Model file for the job. Use its own axes, mm. Face numbers are marked on the shaded views. A direction names the side the tool comes from. Round coordinates to 2 decimals unless told otherwise and drop trailing zeros. Order: outer loops, then holes, each group sorted by start corner. A loop starts at its lowest first (then second) coordinate and runs counter-clockwise, first axis right, second up. Notation, with made-up numbers: (-37, -36) - (12, -36) arc R19 ccw to (12, -13) - close; hole circle Ø6 at (-36, 88.5). An arc over 180 degrees is marked (long way). Put each result on its own line as item: value. Start each with the question number.
Item 1: Saw through at A-A on y = 19.5. State how many separate pieces and enclosed holes the cut face has, plus the area to 3 significant figures.
Item 2: Saw through at D-D on z = 19.3. List the corners of the cut face in (x, y), plus the area to 3 significant figures.
Item 3: Probe probe 1 along Z at (x, y) = (36.5, -3.5); probe 2 along X at (y, z) = (-1.5, -38.7); probe 3 along X at (y, z) = (18.5, -33). List the from-to ranges inside material, lowest first.
Item 4: Mould opens along Z. For the marked faces 1, 2, 3 and 4 say: pulls with the +Z half, pulls with the -Z half, needs draft (parallel to the pull), parting line crosses it, or undercut.
Item 5: Saw through at C-C on x = 3.5. List the corners of the cut face in (y, z).
Item 6: Which spindle directions (+Z, -Z, +X, -X, +Y, -Y) get a long thin tool onto all of the face, cutting with end or side? Do the marked faces 5, 6, 7 and 8. Say none if no direction does.
Item 7: Pin check, flat tips, straight feed: pin 1 Ø2 at (y, z) = (8.5, 15) entering from -X; pin 2 Ø5 at (x, y) = (-63.5, -12) entering from -Z; pin 3 Ø13 at (x, z) = (36, -24.5) entering from +Y. Stop position of each tip, or through.
```python
from build123d import *

# Parameters (mm, degrees)
EXTRUDE_1_DEPTH     = 16
F_1_0MM_1_D         = 3.6
F_1_0MM_2_D         = 3.6
SKETCH_8_W          = 86.7
SKETCH_8_H          = 16
EXTRUDE_2_DEPTH     = 21.2
SKETCH_9_W          = 86.7
SKETCH_9_H          = 10.4
EXTRUDE_3_DEPTH     = 9.7
SKETCH_15_W         = 20.6
SKETCH_15_H         = 2
EXTRUDE_8_DEPTH     = 13.5
SKETCH_16_W         = 20.6
SKETCH_16_H         = 2
EXTRUDE_9_DEPTH     = 10.5
SKETCH_19_W         = 51.4
SKETCH_19_H         = 10.4
EXTRUDE_10_DEPTH    = 50
SKETCH_25_W         = 50
SKETCH_25_H         = 10.4
EXTRUDE_11_DEPTH    = 45
EXTRUDE_12_DEPTH    = 32
CUT_EXTRUDE_1_DEPTH = 5
SKETCH_29_W         = 51.4
SKETCH_29_H         = 10.402970243
EXTRUDE_13_DEPTH    = 40
SKETCH_32_W         = 40
SKETCH_32_H         = 10.402970243
EXTRUDE_14_DEPTH    = 10
SKETCH_33_W         = 40
SKETCH_33_H         = 10.402970243
EXTRUDE_15_DEPTH    = 10
SKETCH_34_R         = 3
EXTRUDE_16_DEPTH    = 18
F_1_0MM_3_D         = 3.6
F_1_0MM_4_D         = 3.6
FILLET_1_R          = 10
FILLET_2_R          = 10
SKETCH_40_W         = 6
SKETCH_40_H         = 4
EXTRUDE_17_DEPTH    = 11.5
SKETCH_42_W         = 6
SKETCH_42_H         = 19.4
EXTRUDE_18_DEPTH    = 2
SKETCH_46_W         = 60.1
SKETCH_46_H         = 4
EXTRUDE_19_DEPTH    = 2


with BuildPart() as part:
    # 草图1 → 凸台-拉伸1 (new body)
    with BuildSketch(Plane.XY):
        Polygon((-21.523113208, 25.59839861), (-42.123113208, 25.59839861), (-42.123113208, 5.59839861), (44.576886792, 5.59839861), (44.576886792, 25.59839861), (23.976886792, 25.59839861), (23.976886792, 13.12839861), (-21.523113208, 13.12839861), align=None)
    extrude_1 = extrude(amount=EXTRUDE_1_DEPTH)

    # Ø1.0mm 暗销孔1 (through all)
    with Locations(Plane(origin=(0, 25.59839861, 0), x_dir=(1, 0, 0), z_dir=(0, 1, 0))):
        with Locations((36.576886792, -8)):
            f_1_0mm_1 = Hole(F_1_0MM_1_D / 2)

    # Ø1.0mm 暗销孔2 (through all)
    with Locations(Plane(origin=(0, 25.59839861, 0), x_dir=(1, 0, 0), z_dir=(0, 1, 0))):
        with Locations((-34.123113208, -8)):
            f_1_0mm_2 = Hole(F_1_0MM_2_D / 2)

    # 草图8 → 凸台-拉伸2 (add)
    with BuildSketch(Plane.XZ.offset(-5.59839861)):
        with Locations((1.226886792, 8)):
            Rectangle(SKETCH_8_W, SKETCH_8_H)
    extrude_2 = extrude(amount=EXTRUDE_2_DEPTH)

    # 草图9 → 凸台-拉伸3 (add)
    with BuildSketch(Plane(origin=(0, 0, 0), x_dir=(-1, 0, 0), z_dir=(0, 0, -1))):
        with Locations((-1.226886792, -10.40160139)):
            Rectangle(SKETCH_9_W, SKETCH_9_H)
    extrude_3 = extrude(amount=EXTRUDE_3_DEPTH)

    # 草图15 → 凸台-拉伸8 (add)
    with BuildSketch(Plane(origin=(0, -5.20160139, 0), x_dir=(1, 0, 0), z_dir=(0, 1, 0))):
        with Locations((-31.823113208, 8.7)):
            Rectangle(SKETCH_15_W, SKETCH_15_H)
    extrude_8 = extrude(amount=EXTRUDE_8_DEPTH)

    # 草图16 → 凸台-拉伸9 (add)
    with BuildSketch(Plane(origin=(0, 0, -9.7), x_dir=(-1, 0, 0), z_dir=(0, 0, -1))):
        with Locations((31.823113208, 7.29839861)):
            Rectangle(SKETCH_16_W, SKETCH_16_H)
    extrude_9 = extrude(amount=-EXTRUDE_9_DEPTH)

    # 镜向20: 凸台-拉伸1, Ø1.0mm 暗销孔1, Ø1.0mm 暗销孔2, 凸台-拉伸2, 凸台-拉伸3, 凸台-拉伸8, 凸台-拉伸9 across plane
    add(extrude_1.mirror(Plane.XY.offset(-9.7)))
    add(f_1_0mm_1.mirror(Plane.XY.offset(-9.7)), mode=Mode.SUBTRACT)
    add(f_1_0mm_2.mirror(Plane.XY.offset(-9.7)), mode=Mode.SUBTRACT)
    add(extrude_2.mirror(Plane.XY.offset(-9.7)))
    add(extrude_3.mirror(Plane.XY.offset(-9.7)))
    add(extrude_8.mirror(Plane.XY.offset(-9.7)))
    add(extrude_9.mirror(Plane.XY.offset(-9.7)))

    # 草图19 → 凸台-拉伸10 (add)
    with BuildSketch(Plane(origin=(44.576886792, 0, 0), x_dir=(0, 0, -1), z_dir=(1, 0, 0))):
        with Locations((9.7, -10.40160139)):
            Rectangle(SKETCH_19_W, SKETCH_19_H)
    extrude(amount=EXTRUDE_10_DEPTH)

    # 草图25 → 凸台-拉伸11 (add)
    with BuildSketch(Plane(origin=(0, 0, -35.4), x_dir=(-1, 0, 0), z_dir=(0, 0, -1))):
        with Locations((-69.576886792, -10.40160139)):
            Rectangle(SKETCH_25_W, SKETCH_25_H)
    extrude(amount=EXTRUDE_11_DEPTH)

    # 草图26 → 凸台-拉伸12 (add)
    with BuildSketch(Plane(origin=(0, -5.20160139, 0), x_dir=(1, 0, 0), z_dir=(0, 1, 0))):
        Polygon((83.176886792, -9), (94.576886792, -9), (94.576886792, -5), (94.576886792, 80.4), (90.576886792, 80.4), (90.576886792, -5), (83.176886792, -5), align=None)
        Polygon((83.176886792, 28), (84.576886792, 28), (84.576886792, 68), (83.176886792, 68), (81.776886792, 68), (81.776886792, 28), align=None)
    extrude(amount=EXTRUDE_12_DEPTH)

    # 草图28 → 切除-拉伸1 (cut)
    with BuildSketch(Plane(origin=(0, -5.20160139, 0), x_dir=(1, 0, 0), z_dir=(0, 1, 0))):
        Polygon((90.576886792, -5), (84.576886792, -5), (82.576886792, -5), (82.576886792, 28), (84.576886792, 28), (84.576886792, 80.4), (90.576886792, 80.4), align=None)
    extrude(amount=-CUT_EXTRUDE_1_DEPTH, mode=Mode.SUBTRACT)

    # 草图29 → 凸台-拉伸13 (add)
    with BuildSketch(Plane.ZY.offset(42.123113208)):
        with Locations((-9.7, -10.400116268)):
            Rectangle(SKETCH_29_W, SKETCH_29_H)
    extrude(amount=EXTRUDE_13_DEPTH)

    # 草图32 → 凸台-拉伸14 (add)
    with BuildSketch(Plane(origin=(0, 0, -35.4), x_dir=(-1, 0, 0), z_dir=(0, 0, -1))):
        with Locations((62.123113208, -10.400116268)):
            Rectangle(SKETCH_32_W, SKETCH_32_H)
    extrude(amount=EXTRUDE_14_DEPTH)

    # 草图33 → 凸台-拉伸15 (add)
    with BuildSketch(Plane.XY.offset(16)):
        with Locations((-62.123113208, -10.400116268)):
            Rectangle(SKETCH_33_W, SKETCH_33_H)
    extrude(amount=EXTRUDE_15_DEPTH)

    # 草图34 → 凸台-拉伸16 (add)
    with BuildSketch(Plane(origin=(0, -5.198631147, 0), x_dir=(1, 0, 0), z_dir=(0, 1, 0))):
        with Locations(Location((-52.123113208, 38.7, 0), (0, 0, 90))):
            Circle(SKETCH_34_R)
        with Locations(Location((-75.123113208, 38.7, 0), (0, 0, 90))):
            Circle(SKETCH_34_R)
        with Locations(Location((-52.123113208, -19.3, 0), (0, 0, 90))):
            Circle(SKETCH_34_R)
        with Locations(Location((-75.123113208, -19.3, 0), (0, 0, 90))):
            Circle(SKETCH_34_R)
    extrude(amount=EXTRUDE_16_DEPTH)

    # Ø1.0mm 暗销孔3 (through all)
    with Locations(Plane(origin=(0, 12.801368853, 0), x_dir=(1, 0, 0), z_dir=(0, 1, 0))):
        with Locations((-52.123113208, 38.7)):
            Hole(F_1_0MM_3_D / 2)

    # Ø1.0mm 暗销孔4 (through all)
    with Locations(Plane(origin=(0, 12.801368853, 0), x_dir=(1, 0, 0), z_dir=(0, 1, 0))):
        with Locations((-52.123113208, -19.3), (-75.123113208, 38.7), (-75.123113208, -19.3)):
            Hole(F_1_0MM_4_D / 2)

    # 圆角1
    fillet_1_edges = [part.edges().sort_by_distance(p)[0] for p in [
        (44.576886792, -10.40160139, -80.4),
        (94.576886792, -10.40160139, 16),
        (-42.123113208, -10.400116268, -45.4),
        (-42.123113208, -10.400116268, 26),
        (-82.123113208, -10.400116268, -45.4),
        (-82.123113208, -10.400116268, 26),
    ]]
    fillet(fillet_1_edges, radius=FILLET_1_R - 0.0001)  # a hair under: the kernel refuses the full size

    # 圆角2
    fillet_2_edges = [part.edges().sort_by_distance(p)[0] for p in [
        (94.576886792, 5.59839861, -80.4),
    ]]
    fillet(fillet_2_edges, radius=FILLET_2_R - 0.0001)  # a hair under: the kernel refuses the full size

    # 草图40 → 凸台-拉伸17 (add)
    with BuildSketch(Plane(origin=(0, -5.20160139, 0), x_dir=(1, 0, 0), z_dir=(0, 1, 0))):
        with Locations((41.576886792, 9.7)):
            Rectangle(SKETCH_40_W, SKETCH_40_H)
    extrude(amount=EXTRUDE_17_DEPTH)

    # 草图42 → 凸台-拉伸18 (add)
    with BuildSketch(Plane(origin=(0, 6.29839861, 0), x_dir=(1, 0, 0), z_dir=(0, 1, 0))):
        with Locations((41.576886792, 9.7)):
            Rectangle(SKETCH_42_W, SKETCH_42_H)
    extrude(amount=EXTRUDE_18_DEPTH)

    # 草图46 → 凸台-拉伸19 (add)
    with BuildSketch(Plane(origin=(0, -5.20160139, 0), x_dir=(1, 0, 0), z_dir=(0, 1, 0))):
        with Locations((8.526886792, 9.7)):
            Rectangle(SKETCH_46_W, SKETCH_46_H)
    extrude(amount=EXTRUDE_19_DEPTH)


solid = part.part
```
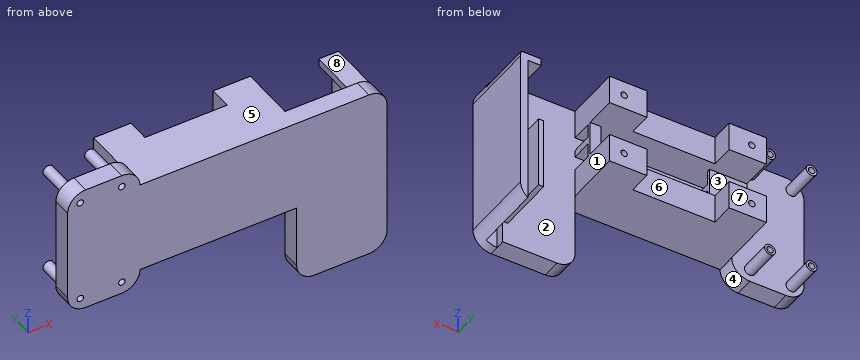
Results found:
1. separate pieces: 6
1. enclosed holes: 4
1. area: 1,760 mm²
2. outline: (-81.56, -15.6) - (-76.92, -15.6) - (-76.92, 12.8) - (-78.12, 12.8) - (-78.12, -5.2) - (-81.56, -5.2) - close; (-73.32, -15.6) - (-53.92, -15.6) - (-53.92, 12.8) - (-55.12, 12.8) - (-55.12, -5.2) - (-72.12, -5.2) - (-72.12, 12.8) - (-73.32, 12.8) - close; (-50.32, -15.6) - (-42.68, -15.6) - (-42.68, -5.2) - (-49.12, -5.2) - (-49.12, 12.8) - (-50.32, 12.8) - close
2. area: 416 mm²
3. probe 1: z = -35.4 to -19.4, -11.7 to -7.7, 0 to 16
3. probe 2: x = -78.12 to -76.92, -73.32 to -72.12, -55.12 to -53.92, -50.32 to -49.12, 81.78 to 84.58, 90.58 to 94.58
3. probe 3: x = -42.12 to -21.52, 23.98 to 44.58, 81.78 to 84.58, 90.58 to 94.58
4. face 1: needs draft
4. face 2: undercut
4. face 3: undercut
4. face 4: pulls with the -Z half
5. outline: (-15.6, -35.4) - (13.13, -35.4) - (13.13, -19.4) - (-5.2, -19.4) - (-5.2, -11.7) - (-3.2, -11.7) - (-3.2, -7.7) - (-5.2, -7.7) - (-5.2, 0) - (13.13, 0) - (13.13, 16) - (-15.6, 16) - close
6. face 5: +Z, +X, +Y, -Y
6. face 6: +Z, -Z, +Y
6. face 7: +Z, -Z, -X, +Y
6. face 8: +Z, +X, +Y
7. pin 1: stops at x = -42.12
7. pin 2: stops at z = -45.4
7. pin 3: stops at y = 25.6
